```python
from build123d import *

# Parameters (mm, degrees)
BOSS_EXTRUDE1_DEPTH        = 5
F_4_5_4_5_DIAMETER_HOLE1_D = 4.5


with BuildPart() as part:
    # Sketch1 → Boss-Extrude1 (new body)
    with BuildSketch(Plane(origin=(0, -74, 0), x_dir=(1, 0, 0), z_dir=(0, 1, 0))):
        with BuildLine():
            Line((9.792858273, -22.023664764), (18.163987442, -36.890703242))
            ThreePointArc((18.163987442, -36.890703242), (25.418865109, -42.641693781), (24.263539525, -33.456250682))
            Line((24.263539525, -33.456250682), (15.892410356, -18.589212204))
            ThreePointArc((15.892410356, -18.589212204), (16.346796769, -18.007963525), (16.757092444, -17.394795929))
            Line((16.757092444, -17.394795929), (18.965700238, -17.831555144))
            ThreePointArc((18.965700238, -17.831555144), (19.514808102, -17.55458812), (19.379909826, -16.954560925))
            Line((19.379909826, -16.954560925), (17.910889228, -15.715657441))
            Line((17.910889228, -15.715657441), (17.664910308, -15.504807423))
            ThreePointArc((17.664910308, -15.504807423), (17.827013037, -15.010242888), (17.963165175, -14.507914341))
            Line((17.963165175, -14.507914341), (20.19864203, -14.240799695))
            ThreePointArc((20.19864203, -14.240799695), (20.635287125, -13.80770474), (20.32157264, -13.278730827))
            Line((20.32157264, -13.278730827), (18.541608797, -12.554415925))
            Line((18.541608797, -12.554415925), (18.242512703, -12.429897308))
            ThreePointArc((18.242512703, -12.429897308), (18.243852713, -11.909445986), (18.218113034, -11.389629824))
            Line((18.218113034, -11.389629824), (20.261634899, -10.444788361))
            ThreePointArc((20.261634899, -10.444788361), (20.543075361, -9.897959827), (20.081253227, -9.491818847))
            Line((20.081253227, -9.491818847), (18.164581401, -9.352993516))
            Line((18.164581401, -9.352993516), (17.841645743, -9.32699505))
            ThreePointArc((17.841645743, -9.32699505), (17.682091866, -8.831602343), (17.496979948, -8.345181793))
            Line((17.496979948, -8.345181793), (19.148512665, -6.815101178))
            ThreePointArc((19.148512665, -6.815101178), (19.247199139, -6.208066452), (18.682475725, -5.964514314))
            Line((18.682475725, -5.964514314), (16.816713109, -6.424767746))
            Line((16.816713109, -6.424767746), (16.501549079, -6.499834341))
            ThreePointArc((16.501549079, -6.499834341), (16.196719559, -6.077992739), (15.870355447, -5.672582033))
            Line((15.870355447, -5.672582033), (16.968235486, -3.707037218))
            ThreePointArc((16.968235486, -3.707037218), (16.874507855, -3.099217089), (16.262162222, -3.042094373))
            Line((16.262162222, -3.042094373), (14.62994266, -4.056373754))
            Line((14.62994266, -4.056373754), (14.353400709, -4.22515737))
            ThreePointArc((14.353400709, -4.22515737), (13.933134384, -3.918159668), (13.497464871, -3.633443231))
            Line((13.497464871, -3.633443231), (13.934224085, -1.424835437))
            ThreePointArc((13.934224085, -1.424835437), (13.657257061, -0.875727573), (13.057229867, -1.010625848))
            Line((13.057229867, -1.010625848), (11.818326382, -2.479646446))
            Line((11.818326382, -2.479646446), (11.607476364, -2.725625367))
            ThreePointArc((11.607476364, -2.725625367), (11.112911829, -2.563522638), (10.610583282, -2.427370499))
            Line((10.610583282, -2.427370499), (10.343468637, -0.191893645))
            ThreePointArc((10.343468637, -0.191893645), (9.910373682, 0.24475145), (9.381399768, -0.068963034))
            Line((9.381399768, -0.068963034), (8.657084866, -1.848926878))
            Line((8.657084866, -1.848926878), (8.532566249, -2.148022972))
            ThreePointArc((8.532566249, -2.148022972), (8.012114927, -2.146682961), (7.492298765, -2.17242264))
            Line((7.492298765, -2.17242264), (6.547457302, -0.128900776))
            ThreePointArc((6.547457302, -0.128900776), (6.000628768, 0.152539686), (5.594487788, -0.309282448))
            Line((5.594487788, -0.309282448), (5.455662457, -2.225954274))
            Line((5.455662457, -2.225954274), (5.429663991, -2.548889932))
            ThreePointArc((5.429663991, -2.548889932), (4.934271284, -2.708443809), (4.447850734, -2.893555727))
            Line((4.447850734, -2.893555727), (2.917770119, -1.24202301))
            ThreePointArc((2.917770119, -1.24202301), (2.310735394, -1.143336536), (2.067183255, -1.70805995))
            Line((2.067183255, -1.70805995), (2.527436687, -3.573822566))
            Line((2.527436687, -3.573822566), (2.602503283, -3.888986596))
            ThreePointArc((2.602503283, -3.888986596), (2.18066168, -4.193816116), (1.775250975, -4.520180228))
            Line((1.775250975, -4.520180228), (-0.19029384, -3.422300189))
            ThreePointArc((-0.19029384, -3.422300189), (-0.79811397, -3.51602782), (-0.855236686, -4.128373453))
            Line((-0.855236686, -4.128373453), (0.159042695, -5.760593015))
            Line((0.159042695, -5.760593015), (0.327826311, -6.037134965))
            ThreePointArc((0.327826311, -6.037134965), (0.020828609, -6.457401291), (-0.263887828, -6.893070804))
            Line((-0.263887828, -6.893070804), (-2.472495622, -6.45631159))
            ThreePointArc((-2.472495622, -6.45631159), (-3.021603486, -6.733278614), (-2.88670521, -7.333305808))
            Line((-2.88670521, -7.333305808), (-1.417684612, -8.572209293))
            Line((-1.417684612, -8.572209293), (-1.171705692, -8.783059311))
            ThreePointArc((-1.171705692, -8.783059311), (-1.333808421, -9.277623846), (-1.469960559, -9.779952393))
            Line((-1.469960559, -9.779952393), (-3.705437414, -10.047067038))
            ThreePointArc((-3.705437414, -10.047067038), (-4.142082509, -10.480161993), (-3.828368024, -11.009135907))
            Line((-3.828368024, -11.009135907), (-2.048404181, -11.733450809))
            Line((-2.048404181, -11.733450809), (-1.749308087, -11.857969426))
            ThreePointArc((-1.749308087, -11.857969426), (-1.750648097, -12.378420747), (-1.724908418, -12.89823691))
            Line((-1.724908418, -12.89823691), (-3.768430283, -13.843078373))
            ThreePointArc((-3.768430283, -13.843078373), (-4.049870744, -14.389906907), (-3.588048611, -14.796047887))
            Line((-3.588048611, -14.796047887), (-1.671376785, -14.934873217))
            Line((-1.671376785, -14.934873217), (-1.348441127, -14.960871684))
            ThreePointArc((-1.348441127, -14.960871684), (-1.188887249, -15.45626439), (-1.003775332, -15.942684941))
            Line((-1.003775332, -15.942684941), (-2.655308048, -17.472765555))
            ThreePointArc((-2.655308048, -17.472765555), (-2.753994523, -18.079800281), (-2.189271109, -18.32335242))
            Line((-2.189271109, -18.32335242), (-0.323508493, -17.863098988))
            Line((-0.323508493, -17.863098988), (-0.008344463, -17.788032392))
            ThreePointArc((-0.008344463, -17.788032392), (0.296485057, -18.209873994), (0.622849169, -18.6152847))
            Line((0.622849169, -18.6152847), (-0.47503087, -20.580829515))
            ThreePointArc((-0.47503087, -20.580829515), (-0.381303238, -21.188649645), (0.231042394, -21.245772361))
            Line((0.231042394, -21.245772361), (1.863261956, -20.23149298))
            Line((1.863261956, -20.23149298), (2.139803907, -20.062709363))
            ThreePointArc((2.139803907, -20.062709363), (2.560070232, -20.369707066), (2.995739745, -20.654423502))
            Line((2.995739745, -20.654423502), (2.558980531, -22.863031297))
            ThreePointArc((2.558980531, -22.863031297), (2.835947555, -23.412139161), (3.43597475, -23.277240885))
            Line((3.43597475, -23.277240885), (4.674878234, -21.808220287))
            Line((4.674878234, -21.808220287), (4.885728252, -21.562241367))
            ThreePointArc((4.885728252, -21.562241367), (5.380292787, -21.724344095), (5.882621334, -21.860496234))
            Line((5.882621334, -21.860496234), (6.149735979, -24.095973089))
            ThreePointArc((6.149735979, -24.095973089), (6.582830934, -24.532618183), (7.111804848, -24.218903699))
            Line((7.111804848, -24.218903699), (7.83611975, -22.438939856))
            Line((7.83611975, -22.438939856), (7.960638367, -22.139843762))
            ThreePointArc((7.960638367, -22.139843762), (8.879420123, -22.123890361), (9.792858273, -22.023664764))
        make_face()
    extrude(amount=-BOSS_EXTRUDE1_DEPTH)

    # Ø4.5 (4.5) Diameter Hole1 (through all)
    with Locations(Plane(origin=(0, -79, 0), x_dir=(-1, 0, 0), z_dir=(0, -1, 0))):
        with Locations((-22.965684708, -38.284870865), (-8.246602308, -12.143933367)):
            Hole(F_4_5_4_5_DIAMETER_HOLE1_D / 2)


solid = part.part
```
Part model, mm, in its own coordinate system. A direction names the side the tool comes from. Round coordinates to 2 decimals unless told otherwise and drop trailing zeros. Loops run counter-clockwise (first coordinate to the right, second up) from the corner with the lowest first, then second, coordinate; pieces in that order, holes last. Notation, with made-up numbers: (13, 82) -> (41, 82) arc R21 cw to (41, 109) -> close; hole circle Ø9 at (44, -2.75). An arc over 180 degrees is marked (long way). Use one line per item in the form item = value. Start each with the question number.
Item 1: Two-plate mould, pull along X, no slides. Class faces 1 (the cylindrical face through (13.7, -76.5, 0.9)), 2 (the flat face through (-1.82, -76.46, 16.7)), 3 (the flat face through (19.136, -76.465, 9.423)): released by +X, released by -X, zero draft, split by the parting line, or undercut.
Item 2: Band-saw the part on B-B (y = -77). Give the number of separate pieces and of enclosed holes in the cut face, plus the area to 3 significant figures.
Item 3: Band-saw the part on A-A (x = 4). List the corners of the cut face in (y, z).
Item 4: Tool access for faces 4 (the cylindrical face through (-1.33, -76.46, 9.27)), 5 (the cylindrical face through (5.37, -76.46, 21.72)), 6 (the flat face through (10.48, -76.46, 1.33)): list every direction of +Z, -Z, +X, -X, +Y, -Y with a clear straight run to the whole face (end or side of a thin tool).
Item 5: Drop flat-ended pins along their axis: pin 1 Ø1.5 at (x, y) = (9, -75.5) entering from -Z; pin 2 Ø3.5 at (x, z) = (8.25, 12.14) entering from +Y. Give the stop position or say it passes through.
Item 6: Drill centre lines: line 1 along X through (y, z) = (-76.25, 23); line 2 along Z through (x, y) = (10, -76.3); line 3 along Z through (x, y) = (-1.5, -77.9). Where is each one in solid material? Low to high.
Item 7: Band-saw the part on C-C (x = 26.5). List the corners of the cut face in (y, z).
Data:
q1.face_1 = undercut
q1.face_2 = released by -X
q1.face_3 = released by +X
q2.separate_pieces = 1
q2.enclosed_holes = 2
q2.area = 530 mm^2
q3.outline = (-79, 2.41) -> (-74, 2.41) -> (-74, 22.61) -> (-79, 22.61) -> close
q4.face_4 = -X, +Y, -Y
q4.face_5 = +Z, +Y, -Y
q4.face_6 = -Z, +Y, -Y
q5.pin_1 = -0.24
q5.pin_2 = through
q6.line_1 = 2.55 to 3.67, 6.02 to 7.61, 10.34 to 18.38
q6.line_2 = -0.22 to 10.73, 13.55 to 22.39
q6.line_3 = 6.65 to 8.5, 9.78 to 14.95, 16.4 to 18.15
q7.outline = (-79, 34.75) -> (-74, 34.75) -> (-74, 41.82) -> (-79, 41.82) -> close
